CAD build for the part. Positions are in the model's coordinates, mm. A direction names the side the tool comes from. Give positions to 0.01 mm unless a question says otherwise; leave off trailing zeros. Write each loop counter-clockwise with the first axis right and the second up, starting at its lowest first coordinate (ties: lowest second). Pieces come first, ordered by that corner, then holes. Notation, with made-up numbers: (82, -8) -> (104, -8) arc R20 ccw to (104, 30) -> close; hole circle Ø8 at (-1.5, 19.25). An arc over 180 degrees is marked (long way). Answer in a Markdown table with one row per item. Add a question column.
```python
from build123d import *

# Parameters (mm, degrees)
SKETCH1_W                          = 250
SKETCH1_H                          = 16
BASE_EXTRUDE_DEPTH                 = 65
ACCESS_START                       = -16
ACCESS_FOR_BLADE_CLAMP_BOLTS_DEPTH = 16
CUT_EXTRUDE2_DEPTH                 = 17
CUT_EXTRUDE3_DEPTH                 = 17
F_1_4_CLEARANCE_HOLE1_D            = 6.5278
CUT_EXTRUDE4_DEPTH                 = 17
CUT_EXTRUDE5_DEPTH                 = 8
F_8_32_TAPPED_HOLE1_D              = 3.4544
F_8_32_TAPPED_HOLE2_D              = 3.4544
F_8_32_TAPPED_HOLE2_DEPTH          = 12.2936
F_8_32_TAPPED_HOLE2_TIP            = 1.037806461
F_8_32_TAPPED_HOLE3_D              = 3.4544
SKETCH20_W                         = 15
SKETCH20_H                         = 30
CUT_EXTRUDE6_DEPTH                 = 8
SKETCH22_W                         = 12.7
SKETCH22_H                         = 11.75
CUT_EXTRUDE8_DEPTH                 = 9.525
CUT_EXTRUDE9_DEPTH                 = 9
FILLET1_R                          = 4.5


with BuildPart() as part:
    # Sketch1 → Base-Extrude (new body)
    with BuildSketch(Plane.XY):
        with Locations((125, 0)):
            Rectangle(SKETCH1_W, SKETCH1_H)
    extrude(amount=BASE_EXTRUDE_DEPTH)

    # Sketch3 → Access for Blade Clamp Bolts (cut)
    with BuildSketch(Plane(origin=(0, 8, 0), x_dir=(-1, 0, 0), z_dir=(0, 1, 0)).offset(ACCESS_START)):
        Polygon((-764.876222455, 30), (-250, 30), (-232, 30), (-214.635668285, 47.364331715), (-212, 65), (-135.896448754, 574.220751675), (-809.679729524, 1352.941618451), (-1438.659503225, 808.720866775), align=None)
    extrude(amount=ACCESS_FOR_BLADE_CLAMP_BOLTS_DEPTH, mode=Mode.SUBTRACT)

    # Sketch6 → Cut-Extrude2 (cut, through all)
    with BuildSketch(Plane(origin=(0, 8, 0), x_dir=(-1, 0, 0), z_dir=(0, 1, 0))):
        with BuildLine():
            Line((-60, 0), (-110, 0))
            Line((-110, 0), (-110, 10))
            Line((-110, 10), (-64, 10))
            ThreePointArc((-64, 10), (-61.171572875, 8.828427125), (-60, 6))
            Line((-60, 6), (-60, 0))
        make_face()
        with BuildLine():
            Line((110, 0), (110, 6))
            ThreePointArc((110, 6), (108.828427125, 8.828427125), (106, 10))
            Line((106, 10), (64, 10))
            ThreePointArc((64, 10), (61.171572875, 8.828427125), (60, 6))
            Line((60, 6), (60, 0))
            Line((60, 0), (110, 0))
        make_face()
    extrude(amount=-CUT_EXTRUDE2_DEPTH, mode=Mode.SUBTRACT)

    # Sketch7 → Cut-Extrude3 (cut, through all)
    with BuildSketch(Plane(origin=(0, 8, 0), x_dir=(-1, 0, 0), z_dir=(0, 1, 0))):
        with BuildLine():
            Line((-217.5, 0), (-110, 0))
            Line((-110, 0), (-110, 10))
            Line((-110, 10), (-175, 10))
            Line((-175, 10), (-175, 16))
            ThreePointArc((-175, 16), (-176.171572875, 18.828427125), (-179, 20))
            Line((-179, 20), (-204, 20))
            Line((-204, 20), (-217.5, 6.5))
            Line((-217.5, 6.5), (-217.5, 5))
            Line((-217.5, 5), (-217.5, 0))
        make_face()
    extrude(amount=-CUT_EXTRUDE3_DEPTH, mode=Mode.SUBTRACT)

    # 1/4 Clearance Hole1 (through all)
    with Locations(Plane(origin=(242.5, 8, 22.5), x_dir=(0, 0, 1), z_dir=(0, 1, 0))):
        with Locations((0, 0), (35, -230), (-16.5, -230), (-15, 0)):
            Hole(F_1_4_CLEARANCE_HOLE1_D / 2)

    # Sketch11 → Cut-Extrude4 (cut, through all)
    with BuildSketch(Plane(origin=(0, 8, 0), x_dir=(-1, 0, 0), z_dir=(0, 1, 0))):
        with BuildLine():
            Line((0, 65), (0, 50))
            Line((0, 50), (-4, 50))
            ThreePointArc((-4, 50), (-5.414213562, 50.585786438), (-6, 52))
            Line((-6, 52), (-6, 65))
            Line((-6, 65), (0, 65))
        make_face()
        with BuildLine():
            Line((0, 0), (-6, 0))
            Line((-6, 0), (-6, 10.5))
            ThreePointArc((-6, 10.5), (-5.414213562, 11.914213562), (-4, 12.5))
            Line((-4, 12.5), (0, 12.5))
            Line((0, 12.5), (0, 0))
        make_face()
    extrude(amount=-CUT_EXTRUDE4_DEPTH, mode=Mode.SUBTRACT)

    # Sketch12 → Cut-Extrude5 (cut)
    with BuildSketch(Plane(origin=(0, 8, 0), x_dir=(-1, 0, 0), z_dir=(0, 1, 0))):
        with BuildLine():
            Line((0, 0), (-20, 0))
            Line((-20, 0), (-20, 8.5))
            ThreePointArc((-20, 8.5), (-18.828427125, 11.328427125), (-16, 12.5))
            Line((-16, 12.5), (0, 12.5))
            Line((0, 12.5), (0, 0))
        make_face()
    extrude(amount=-CUT_EXTRUDE5_DEPTH, mode=Mode.SUBTRACT)

    # #8-32 Tapped Hole1 (through all)
    with Locations(Plane(origin=(56, 8, 26), x_dir=(0, 0, 1), z_dir=(0, 1, 0))):
        with Locations((0, 0)):
            Hole(F_8_32_TAPPED_HOLE1_D / 2)

    # #8-32 Tapped Hole2
    with Locations(Plane.XY.offset(65)):
        with Locations((120, 0)):
            Hole(F_8_32_TAPPED_HOLE2_D / 2, depth=F_8_32_TAPPED_HOLE2_DEPTH)
            with Locations((0, 0, -(F_8_32_TAPPED_HOLE2_DEPTH + F_8_32_TAPPED_HOLE2_TIP / 2))):  # 118° drill point
                Cone(0, F_8_32_TAPPED_HOLE2_D / 2, F_8_32_TAPPED_HOLE2_TIP, mode=Mode.SUBTRACT)

    # #8-32 Tapped Hole3 (through all)
    with Locations(Plane(origin=(0, 8, 0), x_dir=(-1, 0, 0), z_dir=(0, 1, 0))):
        with Locations((-186.5, 26.9)):
            Hole(F_8_32_TAPPED_HOLE3_D / 2)

    # Sketch20 → Cut-Extrude6 (cut)
    with BuildSketch(Plane(origin=(0, 8, 0), x_dir=(-1, 0, 0), z_dir=(0, 1, 0))):
        with Locations((-242.5, 15)):
            Rectangle(SKETCH20_W, SKETCH20_H)
    extrude(amount=-CUT_EXTRUDE6_DEPTH, mode=Mode.SUBTRACT)

    # Sketch22 → Cut-Extrude8 (cut)
    with BuildSketch(Plane(origin=(0, 8, 0), x_dir=(-1, 0, 0), z_dir=(0, 1, 0))):
        with Locations((-186.5, 25.875)):
            Rectangle(SKETCH22_W, SKETCH22_H)
    extrude(amount=-CUT_EXTRUDE8_DEPTH, mode=Mode.SUBTRACT)

    # Sketch23 → Cut-Extrude9 (cut, through all)
    with BuildSketch(Plane(origin=(0, 0, 0), x_dir=(-1, 0, 0), z_dir=(0, 1, 0))):
        with BuildLine():
            Line((-241.35, 16.5), (-250, 16.5))
            Line((-250, 16.5), (-250, 30))
            Line((-250, 30), (-235, 30))
            Line((-235, 30), (-235, 22.85))
            ThreePointArc((-235, 22.85), (-236.859871939, 18.359871939), (-241.35, 16.5))
        make_face()
    extrude(amount=-CUT_EXTRUDE9_DEPTH, mode=Mode.SUBTRACT)

    # Fillet1
    fillet1_edges = [part.edges().sort_by_distance(p)[0] for p in [
        (180.15, 3.2375, 31.75),
        (192.85, 3.2375, 31.75),
    ]]
    fillet(fillet1_edges, radius=FILLET1_R)


solid = part.part
```
Item 1: Slice it at B-B, the plane y = 4.75. State how many separate pieces and enclosed holes the cut face has, then the cut area to 3 significant figures.
Item 2: Which spindle directions (+Z, -Z, +X, -X, +Y, -Y) get a long thin tool onto all of the face, cutting with end or side? Do faces 1 (the face through (245.736, -4.056, 7.925)), 2 (the face through (246, -4, 16.5)), 3 (the face through (20, 4, 4)), 4 (the face through (176.141, 0.112, 18.797)), 5 (the face through (181.503, 3.171, 30.467)). Say none if no direction does.
Item 3: Probe L1, parallel to X at y = 1, z = 26; L2, parallel to X at y = 0.5, z = 27.5; L3, parallel to X at y = -6, z = 7.5. List the from-to ranges inside material, lowest first. Write a range as from..to.
Item 4: Mould opens along X. For faces 6 (the face through (223, 0, 39)), 7 (the face through (116, 8, 32)), 8 (the face through (120, 0, 10)) say: released by +X, released by -X, zero draft, split by the parting line, or undercut.
Item 5: Slice it at A-A, the plane x = 12.5. List the corners of the cut face in (y, z), then the cut area to 3 significant figures.
Item 6: Slice it at D-D, the plane x = 163.5. List the corners of the cut face in (y, z), then the cut area to 3 significant figures.
Item 7: Slice it at C-C, the plane z = 57.5. List the corners of the cut face in (x, y), then the cut area to 3 significant figures.
Item 8: Drop flat-ended pins along their axis: pin 1 Ø6 at (x, z) = (12, 9) entering from +Y; pin 2 Ø6.5 at (y, z) = (3.5, 2.5) entering from +X; pin 3 Ø2 at (x, y) = (114, 1) entering from -Z. Give the stop position or say it passes through.
Answer key:
| question | item | result |
|---|---|---|
| 1 | separate pieces | 1 |
| 1 | enclosed holes | 2 |
| 1 | area | 12,300 mm² |
| 2 | face 1 | +Y, -Y |
| 2 | face 2 | +Z, +X, +Y, -Y |
| 2 | face 3 | -Z, -X, +Y |
| 2 | face 4 | -Z, +Y, -Y |
| 2 | face 5 | -Z, +Y |
| 3 | L1 | x = 0..54.27, 57.73..180.15, 192.85..235 |
| 3 | L2 | x = 0..55.14, 56.86..180.16, 192.84..235 |
| 3 | L3 | x = 6..9.6, 15.4..60.29, 216.5..239.24, 245.76..250 |
| 4 | face 6 | released by +X |
| 4 | face 7 | zero draft |
| 4 | face 8 | undercut |
| 5 | outline | (-8, 0) -> (0, 0) -> (0, 2.74) -> (-8, 2.74) -> close; (-8, 9.26) -> (0, 9.26) -> (0, 12.5) -> (8, 12.5) -> (8, 54.24) -> (-8, 54.24) -> close; (-8, 60.76) -> (8, 60.76) -> (8, 65) -> (-8, 65) -> close |
| 5 | area | 783 mm² |
| 6 | outline | (-8, 10) -> (8, 10) -> (8, 65) -> (-8, 65) -> close |
| 6 | area | 880 mm² |
| 7 | outline | (6, -8) -> (9.24, -8) -> (9.24, 8) -> (6, 8) -> close; (15.76, -8) -> (213.12, -8) -> (213.12, 8) -> (15.76, 8) -> close; hole circle Ø3.45 at (120, 0) |
| 7 | area | 3,200 mm² |
| 8 | pin 1 | stops at y = 0 |
| 8 | pin 2 | stops at x = 235 |
| 8 | pin 3 | stops at z = 10 |
